Answer from the drawing. Dimensions are ordinates in mm from the lowest x, y and z of the part. Give positions to 0.01 mm unless a question says otherwise; leave off trailing zeros. Loops run counter-clockwise (first coordinate to the right, second up) from the corner with the lowest first, then second, coordinate; pieces in that order, holes last. Notation, with made-up numbers: (-22.75, 7.25) - (18.25, 7.25) arc R31 cw to (18.25, 40.25) - close; hole circle Ø1 at (62, -8.75). An arc over 180 degrees is marked (long way). One line per question, with ' | ' between items. Start each with the question number.
1. For a pull along Y with two mould halves and no side action, classify the marked faces 1, 2, 3 and 4 as released by +Y, released by -Y, zero draft, split by the parting line, or undercut.
2. Section A-A (y = 10) is taken. Determine the outline of the cut face in (x, z) (1 decimal).
3. Section B-B (x = 51) is taken. Determine the outline of the cut face in (y, z) (1 decimal), plus the area to 3 significant figures.
4. Each of these flat-tipped pins is pushed along its axis until it touches: pin 1 (12 mm diameter, centred on x = 7, y = 26.5, fed in from +Z); pin 2 (2.5 mm diameter, centred on y = 20, z = 41.5, fed in from -X); pin 3 (7 mm diameter, centred on x = 51, y = 10, fed in from +Z); pin 4 (8 mm diameter, centred on x = 55, y = 26.5, fed in from -Z) (1 decimal). Where does it stop, or does it pass through?
5. Find the intervals of material crossed by line 1 (Y direction, x = 51, z = 37.75); line 2 (Y direction, x = 51, z = 44.2); line 3 (X direction, y = 10, z = 40.75) (1 decimal), in increasing order.
6. Section C-C (z = 41) is taken. Determine the outline of the cut face in (x, y), plus the area to 3 significant figures.
7. Section D-D (y = 17) is taken. Determine the outline of the cut face in (x, z) (1 decimal).
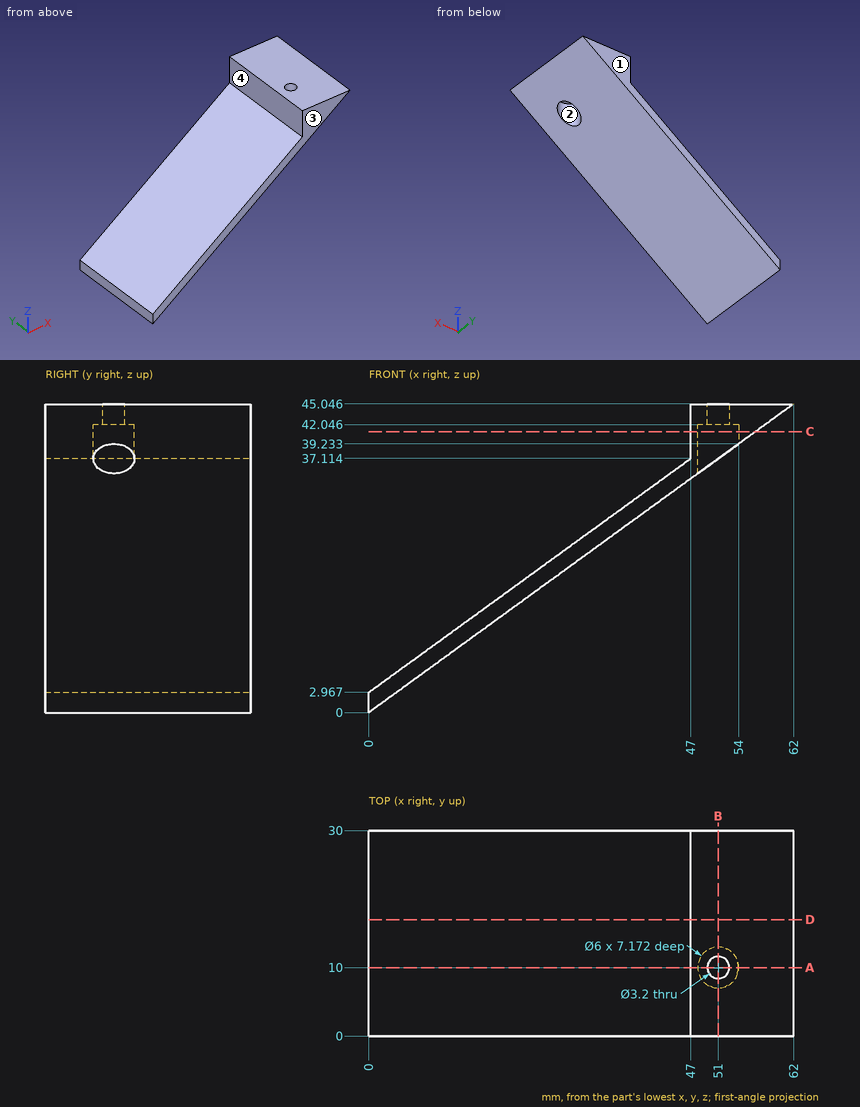
Conclusion:
1) face 1: released by +Y | face 2: undercut | face 3: released by -Y | face 4: zero draft
2) outline: (0, 0) - (48, 34.9) - (48, 42) - (49.4, 42) - (49.4, 45) - (47, 45) - (47, 37.1) - (0, 3) - close; (52.6, 42) - (54, 42) - (54, 39.2) - (62, 45) - (52.6, 45) - close
3) outline: (0, 37.1) - (7, 37.1) - (7, 42) - (8.4, 42) - (8.4, 45) - (0, 45) - close; (11.6, 42) - (13, 42) - (13, 37.1) - (30, 37.1) - (30, 45) - (11.6, 45) - close | area: 200 mm²
4) pin 1: z = 12.41 | pin 2: x = 47 | pin 3: z = 45.05 | pin 4: z = 37.1
5) line 1: 0 to 7, 13 to 30 | line 2: 0 to 8.4, 11.6 to 30 | line 3: 47 to 48, 54 to 56.1
6) outline: (47, 0) - (56.43, 0) - (56.43, 30) - (47, 30) - close; hole circle Ø6 at (51, 10) | area: 255 mm²
7) outline: (0, 0) - (62, 45) - (47, 45) - (47, 37.1) - (0, 3) - close
